from build123d import *
from build123d.topology import SkipClean

# Parameters (mm, degrees)
CROQUIS1_R              = 1.5
SALIENTE_EXTRUIR1_DEPTH = 15
CROQUIS2_R              = 2.5
CORTAR_EXTRUIR1_DEPTH   = 20
CORTAR_EXTRUIR2_START   = -26
CROQUIS4_W              = 5.5
CROQUIS4_H              = 5
CORTAR_EXTRUIR2_DEPTH   = 26


with BuildPart() as part:
    # Croquis1 → Saliente-Extruir1 (new body)
    with BuildSketch(Plane.XY):
        with BuildLine():
            Line((11.25, 17.1), (11.25, 14.1))
            Line((11.25, 14.1), (23.75, 14.1))
            Line((23.75, 14.1), (23.75, 11.1))
            Line((23.75, 11.1), (11.25, 11.1))
            Line((11.25, 11.1), (11.25, 5.1))
            Line((11.25, 5.1), (23.75, 5.1))
            Line((23.75, 5.1), (23.75, 2.1))
            Line((23.75, 2.1), (11.25, 2.1))
            Line((11.25, 2.1), (11.25, -0.9))
            Line((11.25, -0.9), (5.75, -0.9))
            ThreePointArc((5.75, -0.9), (0.800252532, 1.150252532), (-1.25, 6.1))
            Line((-1.25, 6.1), (-1.25, 10.1))
            ThreePointArc((-1.25, 10.1), (0.800252532, 15.049747468), (5.75, 17.1))
            Line((5.75, 17.1), (11.25, 17.1))
        make_face()
        with Locations((3.75, 8.1)):
            Circle(CROQUIS1_R, mode=Mode.SUBTRACT)
    extrude(amount=SALIENTE_EXTRUIR1_DEPTH)

    # Croquis2 → Cortar-Extruir1 (cut)
    with BuildSketch(Plane(origin=(0, 0, 0), x_dir=(1, 0, 0), z_dir=(0, 1, 0))):
        with Locations((17.5, -7.5)):
            Circle(CROQUIS2_R)
        with BuildLine():
            Line((17.5, -1.25), (11.25, 0))
            Line((11.25, 0), (11.126279301, 1.868603497))
            Line((11.126279301, 1.868603497), (29.663453957, 1.868603497))
            Line((29.663453957, 1.868603497), (29.663453957, -17.961269996))
            Line((29.663453957, -17.961269996), (11.25, -17.961269996))
            Line((11.25, -17.961269996), (11.25, -15))
            Line((11.25, -15), (17.5, -13.75))
            ThreePointArc((17.5, -13.75), (23.75, -7.5), (17.5, -1.25))
        make_face()
    extrude(amount=CORTAR_EXTRUIR1_DEPTH, mode=Mode.SUBTRACT)

    # Croquis4 → Cortar-Extruir2 (cut)
    with SkipClean():  # the faces are left unmerged after this step: merging them gives an invalid solid
        with BuildSketch(Plane(origin=(0, 17.1, 0), x_dir=(1, 0, 0), z_dir=(0, 1, 0)).offset(CORTAR_EXTRUIR2_START)):
            with BuildLine():
                Line((-4.389645589, -5), (5.75, -5))
                Line((5.75, -5), (5.75, 0))
                Line((5.75, 0), (11.25, 0))
                Line((11.25, 0), (11.25, -5))
                Line((11.25, -5), (12.730653795, -3.460713334))
                ThreePointArc((12.730653795, -3.460713334), (12.995627449, -3.167203221), (13.278631189, -2.891036411))
                ThreePointArc((13.278631189, -2.891036411), (15.2354385, -1.674687887), (17.5, -1.25))
                Line((17.5, -1.25), (17.5, 1.887707064))
                Line((17.5, 1.887707064), (-4.389645589, 1.887707064))
                Line((-4.389645589, 1.887707064), (-4.389645589, -5))
            make_face()
            with Locations((8.5, -2.5)):
                Rectangle(CROQUIS4_W, CROQUIS4_H)
            with BuildLine():
                Line((5.75, -10), (-4.389645589, -10))
                Line((-4.389645589, -10), (-4.389645589, -16.45653889))
                Line((-4.389645589, -16.45653889), (17.5, -16.45653889))
                Line((17.5, -16.45653889), (17.5, -13.75))
                ThreePointArc((17.5, -13.75), (14.878268112, -13.173536984), (12.740162296, -11.550487011))
                Line((12.740162296, -11.550487011), (11.25, -10))
                Line((11.25, -10), (11.25, -15))
                Line((11.25, -15), (5.75, -15))
                Line((5.75, -15), (5.75, -10))
            make_face()
            with Locations((8.5, -12.5)):
                Rectangle(CROQUIS4_W, CROQUIS4_H)
        extrude(amount=CORTAR_EXTRUIR2_DEPTH, mode=Mode.SUBTRACT)


solid = part.part
Verification items for the finished model (mm, model axes). A direction names the side the tool comes from. Coordinates: 2 decimals unless noted, no trailing zeros. Order: outer loops, then holes, each group sorted by start corner. A loop starts at its lowest first (then second) coordinate and runs counter-clockwise, first axis right, second up.
1. Release check for a two-part mould opening along Z. For faces 6 (the face through (11.98, 12.58, 4.24)), 7 (the face through (15, 12.6, 7.4)), 8 (the face through (11.25, 1, 7)) record: +Z half, -Z half, draft (parallel to the pull), parting line (faces both ways), or undercut.
Results found:
face 6: -Z half
face 7: undercut
face 8: draft
2. Sectioned sample at A-A, the plane z = 7.5. Record the cut outline in (x, y), and give its area (3 significant figures).
Results found:
outline: (-1.25, 6.1) arc R7 ccw to (5.75, -0.9) - (11.25, -0.9) - (11.25, 2.1) - (15, 2.1) - (15, 5.1) - (11.25, 5.1) - (11.25, 11.1) - (15, 11.1) - (15, 14.1) - (11.25, 14.1) - (11.25, 17.1) - (5.75, 17.1) arc R7 ccw to (-1.25, 10.1) - close; (20, 2.1) - (23.75, 2.1) - (23.75, 5.1) - (20, 5.1) - close; (20, 11.1) - (23.75, 11.1) - (23.75, 14.1) - (20, 14.1) - close; hole circle Ø3 at (3.75, 8.1)
area: 242 mm2
3. Scan lines: line 1 (Z direction, x = 17.5, y = 4.05); line 2 (X direction, y = 8.1, z = 9); line 3 (Y direction, x = 14.5, z = 7). Record each from-to range of solid material in increasing order.
Results found:
line 1: z = 1.25 to 5, 10 to 13.75
line 2: x = -1.25 to 2.25, 5.25 to 11.25
line 3: y = 2.1 to 5.1, 11.1 to 14.1
4. Sectioned sample at C-C, the plane y = 8.1. Record the cut outline in (x, z).
Results found:
outline: (-1.25, 5) - (2.25, 5) - (2.25, 10) - (-1.25, 10) - close; (5.25, 5) - (11.25, 5) - (11.25, 10) - (5.25, 10) - close
5. Go/stop test with flat-tipped pins: pin 1 Ø8 at (x, y) = (20.5, 5.5) entering from +Z; pin 2 Ø6.5 at (x, z) = (17.5, 7.5) entering from +Y; pin 3 Ø4 at (x, y) = (5.5, 10) entering from -Z; pin 4 Ø1 at (x, y) = (20, 12.5) entering from +Z. Record where each tip stops, or that it passes through.
Results found:
pin 1: stops at z = 13.75
pin 2: stops at y = 14.1
pin 3: stops at z = 5
pin 4: stops at z = 13.42
6. Set-up check for faces 1 (the face through (17.6, 2.1, 10.2)), 2 (the face through (6, 8, 10)), 3 (the face through (11.25, 8, 7)), 4 (the face through (6, 8, 5)), 5 (the face through (11.25, 16, 7)): record each of +Z, -Z, +X, -X, +Y, -Y from which the full face is reachable in a straight line by a thin tool's end or side.
Results found:
face 1: +Z, -Z, +X, -Y
face 2: +Z, -X, +Y, -Y
face 3: +Z, -Z, +X
face 4: -Z, -X, +Y, -Y
face 5: +Z, -Z, +X, +Y
7. Sectioned sample at B-B, the plane x = 13.75. Record the cut outline in (y, z).
Results found:
outline: (2.1, 2.5) - (5.1, 2.5) - (5.1, 12.5) - (2.1, 12.5) - close; (11.1, 2.5) - (14.1, 2.5) - (14.1, 12.5) - (11.1, 12.5) - close
8. Sectioned sample at D-D, the plane x = 9.5. Record the cut outline in (y, z), and give its area (3 significant figures).
Results found:
outline: (-0.9, 5) - (17.1, 5) - (17.1, 10) - (-0.9, 10) - close
area: 90.0 mm2
